```python
from build123d import *

# Parameters (mm, degrees)
F0_W     = 412
F0_H     = 1100
F1_DEPTH = 18
F2_W     = 350
F2_H     = 80
F3_DEPTH = 25
F4_R     = 2.5
F5_DEPTH = 15


with BuildPart() as f1:
    # F0 (on Top) → F1 (new body)
    with BuildSketch(Plane.XY):
        with Locations((3.552631, 303.48327)):
            Rectangle(F0_W, F0_H)
    extrude(amount=F1_DEPTH)

    # F2 (on face) → F3 (cut)
    with BuildSketch(Plane.XY.offset(18)):
        with Locations((12.552631, -206.51673)):
            Rectangle(F2_W, F2_H)
    extrude(amount=-F3_DEPTH, mode=Mode.SUBTRACT)

    # F4 (on face) → F5 (cut)
    with BuildSketch(Plane.XY.offset(18)):
        with Locations((194.552631, 778.48327)):
            Circle(F4_R)
        with Locations((174.552631, 778.48327)):
            Circle(F4_R)
        with Locations((-152.447369, 818.48327)):
            Circle(F4_R)
        with Locations((-152.447369, 838.48327)):
            Circle(F4_R)
        with Locations((194.552631, -121.51673)):
            Circle(F4_R)
        with Locations((174.552631, -121.51673)):
            Circle(F4_R)
        with Locations((-152.447369, 520.48327)):
            Circle(F4_R)
        with Locations((-152.447369, 500.48327)):
            Circle(F4_R)
    extrude(amount=-F5_DEPTH, mode=Mode.SUBTRACT)


solid = f1.part
```
Part model, mm, in its own coordinate system. A direction names the side the tool comes from. Coordinates: 2 decimals unless noted, no trailing zeros. Order: outer loops, then holes, each group sorted by start corner. A loop starts at its lowest first (then second) coordinate and runs counter-clockwise, first axis right, second up. Notation, with made-up numbers: (86.25, 50.25) - (144.25, 50.25) arc R25 ccw to (144.25, 81.25) - close; hole circle Ø11 at (44, -31). An arc over 180 degrees is marked (long way). Return JSON: item names as keys, results as strings. Group by question number.
Item 1: Drill centre line: probe 1 along Y at (x, z) = (178.5, 6.25). Where is it in solid material? Low to high. Write a range as from..to.
Item 2: Cut at A-A (z = 12.25). State how many separate pieces and enclosed holes the cut face has, plus the area to 3 significant figures.
Item 3: Pull direction X, two halves, no side cores. Call faces 1 (the face through (209.553, 296, 9)), 2 (the face through (10, -166.517, 9)), 3 (the face through (1, 853.483, 9)): pulls with the +X half, pulls with the -X half, needs draft (parallel to the pull), parting line crosses it, or undercut.
Item 4: Pin check, flat tips, straight feed: pin 1 (4 mm diameter, centred on x = -152.45, y = 818.48, fed in from +Z); pin 2 (2 mm diameter, centred on x = -18.5, z = 12, fed in from -Y). Stop position of each tip, or through.
Item 5: Which spindle directions (+Z, -Z, +X, -X, +Y, -Y) get a long thin tool onto all of the face, cutting with end or side? Do faces 4 (the face through (-162.447, -207, 9)), 5 (the face through (198, -246.517, 9)). Say none if no direction does.
Item 6: Cut at B-B (x = 77). List the corners of the cut face in (y, z), plus the area to 3 significant figures.
Check values:
{
 "1": {"probe 1": "y = -166.52..853.48"},
 "2": {"separate pieces": "1", "enclosed holes": "8", "area": "425,000 mm2"},
 "3": {"face 1": "pulls with the +X half", "face 2": "undercut", "face 3": "needs draft"},
 "4": {"pin 1": "stops at z = 3", "pin 2": "stops at y = -166.52"},
 "5": {"face 4": "+Z, -Z, -Y", "face 5": "+Z, -Z, +X, -X, -Y"},
 "6": {"outline": "(-166.52, 0) - (853.48, 0) - (853.48, 18) - (-166.52, 18) - close", "area": "18,400 mm2"}
}
